Part model, mm, in its own coordinate system. Coordinates: 2 decimals unless noted, no trailing zeros. Loops run counter-clockwise (first coordinate to the right, second up) from the corner with the lowest first, then second, coordinate; pieces in that order, holes last. Notation, with made-up numbers: M 59.25,-26.5 L 76.25,-26.5 A31 cw 76.25,2.5 Z; hole C -2,-10.5 d3. An arc over 180 degrees is marked long. Answer as a JSON object with one key per item and string values. Group by question number.
1. Saw through at B-B on z = -9.5. Write the cut outline in (x, y).
2. Drill centre lines: L1, parallel to Y at x = 0.1, z = -6; L2, parallel to Y at x = 0.2, z = -17; L3, parallel to Z at x = 0.45, y = 10. Where is each one in solid material? Low to high.
3. Saw through at C-C on x = 0.1. Write the cut outline in (y, z).
4. Drop a flat-ended pin along its axis: pin 1 Ø4 at (y, z) = (-18.5, -11.5) entering from -X. Give the stop position or say it passes through.
from build123d import *

# Parameters (mm, degrees)
F1_DEPTH = 0.5
F2_SIZE2 = 1.49999
F2_SIZE  = 0.49999


# Not quite as in the source:
# - a fillet or chamfer is up to 0.001 mm smaller than in the source, because OpenCascade refuses the exact size


with BuildPart() as f1:
    # F0 (on Right) → F1 (new body)
    with BuildSketch(Plane.YZ):
        Polygon((15, 0), (-15, 0), (-23.7177978871, -18), (6.2822021129, -18), align=None)
    extrude(amount=F1_DEPTH)

    # F2 (size 0.5 and 1.5 in the source; OpenCascade refuses exactly that, so slightly less here)
    f2_edges = [f1.edges().sort_by_distance(p)[0] for p in [
        (0.5, -8.717798, -18),
    ]]
    f2_side = f1.faces().sort_by_distance((0.25, -8.717798, -18))[0]
    chamfer(f2_edges, length=F2_SIZE, length2=F2_SIZE2, reference=f2_side)


solid = f1.part
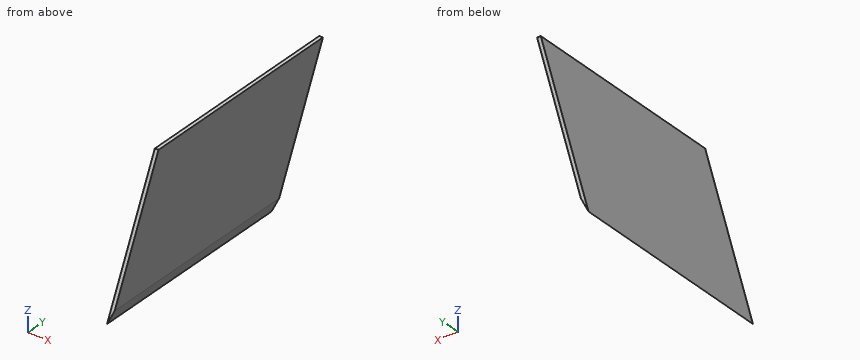
Outcome:
{
 "1": {"outline": "M 0,-19.6 L 0.5,-19.6 L 0.5,10.4 L 0,10.4 Z"},
 "2": {"L1": "y = -17.91 to 12.09", "L2": "y = -23.23 to 6.77", "L3": "z = -10.32 to 0"},
 "3": {"outline": "M -23.57,-17.7 L 6.43,-17.7 L 15,0 L -15,0 Z"},
 "4": {"pin 1": "stops at x = 0"}
}
